Here's how the part is built. I have some questions about the finished solid (model axes, mm). Face numbers are marked on the shaded views. A direction names the side the tool comes from. Give positions to 0.01 mm unless a question says otherwise; leave off trailing zeros. Loops run counter-clockwise (first coordinate to the right, second up) from the corner with the lowest first, then second, coordinate; pieces in that order, holes last.
Q1. We'd pull the mould along Y, two halves only. Please class the marked faces 1, 2 and 3: +Y half, -Y half, draft (parallel to the pull), parting line (faces both ways), or undercut.
Q2. If we section it at C-C (y = 6.75): Please give me the cut outline in (x, z).
Q3. If we section it at B-B (x = -22): Please give me the cut outline in (y, z).
Q4. If we section it at D-D (x = 4.5): Please give me the cut outline in (y, z), plus the area to 3 significant figures.
Q5. Will these pins go through, and if not, where does the flat tip stop? P1, Ø2.5, axis at x = 14.23, y = 1.48, coming from the +Z side; P2, Ø8, axis at x = 6.53, y = -2.82, coming from the -Z side.
Q6. I need wall thicknesses on line 1 (X direction, y = 1.5, z = 4); line 2 (X direction, y = 2.5, z = 5); line 3 (Y direction, x = -5, z = 4). Which ranges of each line are inside material? Lowest first, please.
Q7. For the marked faces 4, 5 and 6, which set-ups out of +Z, -Z, +X, -X, +Y, -Y let a thin tool reach every point of the face, with its end or its side?
Q8. If we section it at A-A (z = 4.5): Please give me the cut outline in (x, y), plus the area to 3 significant figures.
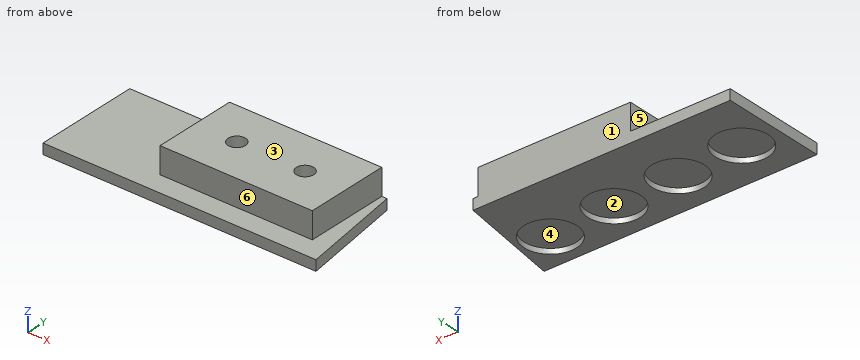
from build123d import *

# Parameters (mm, degrees)
F1_DEPTH = 2
F2_R     = 5
F3_DEPTH = 1
F4_W     = 29
F4_H     = 16
F5_DEPTH = 5
F7_D     = 3.3
F7_DEPTH = 5
F7_TIP   = 0.9914200214


with BuildPart() as f1:
    # F0 (on Top) → F1 (new body)
    with BuildSketch(Plane.XY):
        Polygon((23.2306010574, 9.4812756346), (-25.7693989426, 9.4812756346), (-25.7693989426, -10.5187243654), (26.2306010574, -10.5187243654), align=None)
    extrude(amount=F1_DEPTH)

    # F2 (on face) → F3 (cut)
    with BuildSketch(Plane(origin=(0, 0, 0), x_dir=(1, 0, 0), z_dir=(0, 0, -1))):
        with Locations((19.2306010574, 3.5187243654)):
            Circle(F2_R)
        with Locations((6.5306010574, 2.8187243654)):
            Circle(F2_R)
        with Locations((-6.1693989426, 2.2187243654)):
            Circle(F2_R)
        with Locations((-18.8693989426, 1.5187243654)):
            Circle(F2_R)
    extrude(amount=-F3_DEPTH, mode=Mode.SUBTRACT)

    # F4 (on face) → F5 (join)
    with BuildSketch(Plane.XY.offset(2)):
        with Locations((7.7306010574, 1.4812756346)):
            Rectangle(F4_W, F4_H)
    extrude(amount=F5_DEPTH)

    # F7
    with Locations(Plane.XY.offset(7)):
        with Locations((1.2306010574, 1.4812756346), (14.2306010574, 1.4812756346)):
            Hole(F7_D / 2, depth=F7_DEPTH)
            with Locations((0, 0, -(F7_DEPTH + F7_TIP / 2))):  # 118° drill point
                Cone(0, F7_D / 2, F7_TIP, mode=Mode.SUBTRACT)


solid = f1.part
Check sheet entries:
1. face 1: +Y half
1. face 2: undercut
1. face 3: draft
2. outline: (-25.77, 0) - (23.64, 0) - (23.64, 2) - (22.23, 2) - (22.23, 7) - (-6.77, 7) - (-6.77, 2) - (-25.77, 2) - close
3. outline: (-10.52, 0) - (-5.42, 0) - (-5.42, 1) - (2.38, 1) - (2.38, 0) - (9.48, 0) - (9.48, 2) - (-10.52, 2) - close
4. outline: (-10.52, 0) - (-7.39, 0) - (-7.39, 1) - (1.75, 1) - (1.75, 0) - (9.48, 0) - (9.48, 7) - (-6.52, 7) - (-6.52, 2) - (-10.52, 2) - close
4. area: 111 mm2
5. P1: stops at z = 1.76
5. P2: stops at z = 1
6. line 1: x = -6.77 to -0.42, 2.88 to 12.58, 15.88 to 22.23
6. line 2: x = -6.77 to -0.07, 2.53 to 12.93, 15.53 to 22.23
6. line 3: y = -6.52 to 9.48
7. face 4: -Z
7. face 5: +Z, -X, +Y, -Y
7. face 6: +Z, +X, -X, -Y
8. outline: (-6.77, -6.52) - (22.23, -6.52) - (22.23, 9.48) - (-6.77, 9.48) - close; hole circle Ø3.3 at (1.23, 1.48); hole circle Ø3.3 at (14.23, 1.48)
8. area: 447 mm2
